Part print with two shaded views. Sizes in mm from the minimum x, y, z corner. A direction names the side the tool comes from. Give positions to 0.01 mm unless a question says otherwise; leave off trailing zeros. Order: outer loops, then holes, each group sorted by start corner. A loop starts at its lowest first (then second) coordinate and runs counter-clockwise, first axis right, second up. Notation, with made-up numbers: (58, 37.25) -> (115, 37.25) arc R14 ccw to (115, 53.25) -> close; hole circle Ø8 at (-21.75, 21). An arc over 180 degrees is marked (long way). Answer as CSV lines item,"result".
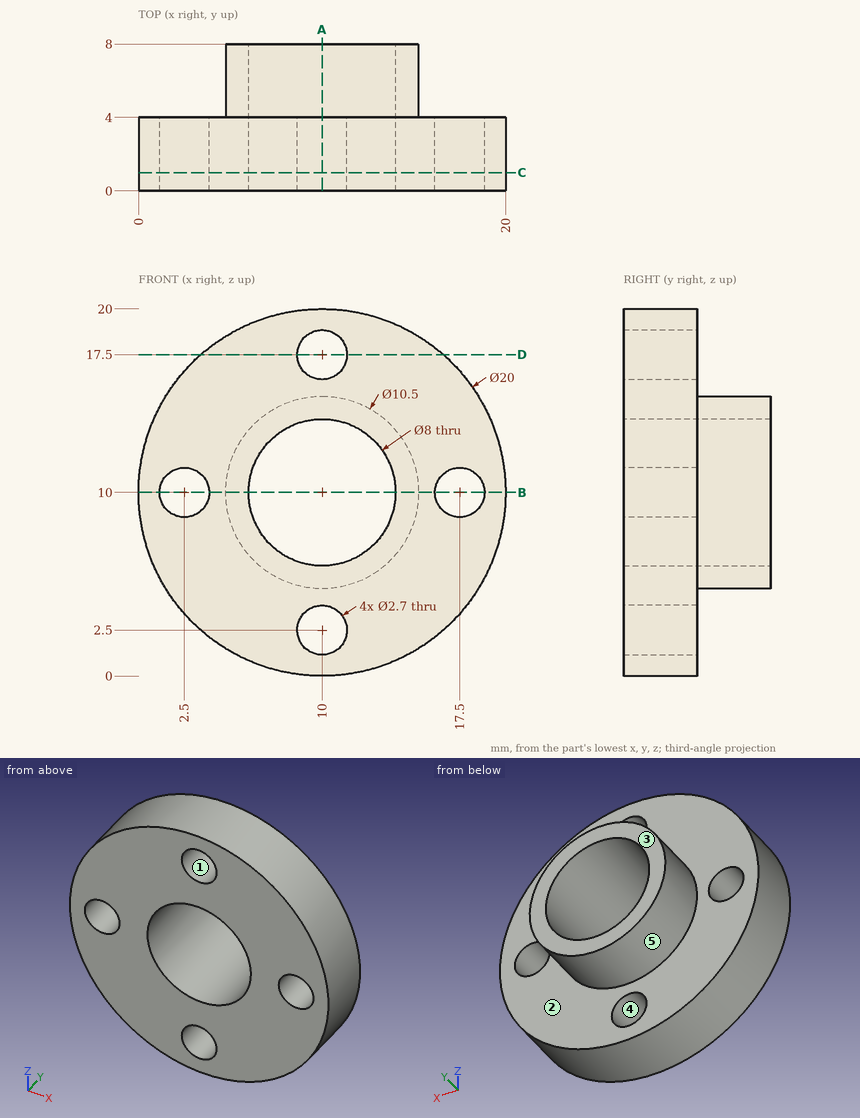
1) Band-saw the part on B-B, the plane z = 10. Write the cut outline in (x, y).
Data:
outline,"(0, 0) -> (1.15, 0) -> (1.15, 4) -> (0, 4) -> close; (3.85, 0) -> (6, 0) -> (6, 8) -> (4.75, 8) -> (4.75, 4) -> (3.85, 4) -> close; (14, 0) -> (16.15, 0) -> (16.15, 4) -> (15.25, 4) -> (15.25, 8) -> (14, 8) -> close; (18.85, 0) -> (20, 0) -> (20, 4) -> (18.85, 4) -> close"
2) Band-saw the part on C-C, the plane y = 1. Write the cut outline in (x, z), then the cut area to 3 significant figures.
Data:
outline,"circle Ø20 at (10, 10); hole circle Ø2.7 at (2.5, 10); hole circle Ø8 at (10, 10); hole circle Ø2.7 at (10, 2.5); hole circle Ø2.7 at (10, 17.5); hole circle Ø2.7 at (17.5, 10)"
area,"241 mm2"
3) Which spindle directions (+Z, -Z, +X, -X, +Y, -Y) get a long thin tool onto all of the face, cutting with end or side? Do the marked faces 1 and 2. Say none if no direction does.
Data:
face 1,"+Y, -Y"
face 2,"+Y"
4) Band-saw the part on A-A, the plane x = 10. Write the cut outline in (y, z), then the cut area to 3 significant figures.
Data:
outline,"(0, 0) -> (4, 0) -> (4, 1.15) -> (0, 1.15) -> close; (0, 3.85) -> (4, 3.85) -> (4, 4.75) -> (8, 4.75) -> (8, 6) -> (0, 6) -> close; (0, 14) -> (8, 14) -> (8, 15.25) -> (4, 15.25) -> (4, 16.15) -> (0, 16.15) -> close; (0, 18.85) -> (4, 18.85) -> (4, 20) -> (0, 20) -> close"
area,"36.4 mm2"
5) Pull direction X, two halves, no side cores. Call the marked faces 3, 4 and 5: pulls with the +X half, pulls with the -X half, needs draft (parallel to the pull), parting line crosses it, or undercut.
Data:
face 3,"needs draft"
face 4,"undercut"
face 5,"parting line crosses it"
6) Pin check, flat tips, straight feed: P1, Ø7, axis at x = 10, z = 10, coming from the +Y side; P2, Ø3, axis at x = 10, z = 2.5, coming from the +Y side; P3, Ø4, axis at x = 5.5, y = 5, coming from the +Z side; P4, Ø4, axis at y = 6.5, z = 13, coming from the -X side. Stop position of each tip, or through.
Data:
P1,"passes through"
P2,"stops at y = 4"
P3,"stops at z = 19.61"
P4,"stops at x = 4.85"
7) Band-saw the part on D-D, the plane z = 17.5. Write the cut outline in (x, y).
Data:
outline,"(3.39, 0) -> (8.65, 0) -> (8.65, 4) -> (3.39, 4) -> close; (11.35, 0) -> (16.61, 0) -> (16.61, 4) -> (11.35, 4) -> close"
8) Wall check: line 1 along X through (y, z) = (2.5, 10); line 2 along Y through (x, z) = (6.25, 16.5); line 3 along Z through (x, y) = (9.25, 1.75). Give the ranges that are in metal, low to high. Write a range as [from, to].
Data:
line 1,"x = [0, 1.15], [3.85, 6], [14, 16.15], [18.85, 20]"
line 2,"y = [0, 4]"
line 3,"z = [0.03, 1.38], [3.62, 6.07], [13.93, 16.38], [18.62, 19.97]"
